Verification items for the finished model (mm, model axes). Face numbers are marked on the shaded views. Coordinates: 2 decimals unless noted, no trailing zeros. Write each loop counter-clockwise with the first axis right and the second up, starting at its lowest first coordinate (ties: lowest second). Pieces come first, ordered by that corner, then holes. Notation, with made-up numbers: M -23.5,65.25 L 32.5,65.25 A14 cw 32.5,80.25 Z; hole C -37.75,89 d9. An arc over 180 degrees is marked long. Answer in a Markdown table with one row per item.
Autodesk Fusion 360 part; units mm, degrees
sketch "Esboço1" plane through (0, 0, 0) normal (0, 1, 0) x (1, 0, 0)
  circle A0 centre (0, 0) radius 7.25
  dimension "d1" = 14.5
extrude "Extrusão1" add sketch "Esboço1" along normal blind 1
sketch "Esboço2" plane through (0, 1, 0) normal (0, 1, 0) x (-1, 0, 0)
  circle A0 centre (0, 0) radius 7.25
  circle A1 centre (0, 0) radius 6.8
  circle A2 centre (0, 0) radius 5.3
  dimension "d4" = 13.6
  dimension "d5" = -1.5
extrude "Extrusão2" add sketch "Esboço2" along normal blind 5 contours A1
sketch "Esboço3" plane through (0, 0, 0) normal (0, 0, 1) x (1, 0, 0)
  line L0 (6.8, 6) -> (6.8, 4)
  line L1 (6.8, 5) -> (6.9, 5)
  line L2 (6.9, 5) -> (6.8, 4)
  line L3 (6.9, 5) -> (6.8, 6)
revolve "Revolucionar1" add sketch "Esboço3" angle 360 about axis through (0, 1.75, 0) along (0, 1, 0)
fillet "Arredondamento1" radius 0.55 1 edges at (6.3398, 6, -2.459)
fillet "Arredondamento2" radius 0.55 1 edges at (4.9413, 6, 1.9166)
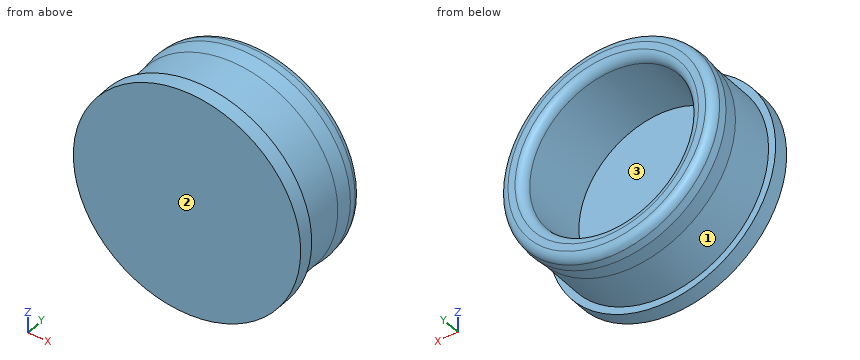
1) Sectioned sample at A-A (x = 0). Record the cut outline in (y, z), then the cut area to 3 significant figures.
Response values:
| item | result |
|---|---|
| outline | M 0,-7.25 L 1,-7.25 L 1,-6.8 L 4,-6.8 L 5,-6.9 L 5.5,-6.85 A0.55 ccw 6,-6.3 L 6,-5.85 A0.55 ccw 5.45,-5.3 L 1,-5.3 L 1,5.3 L 5.45,5.3 A0.55 ccw 6,5.85 L 6,6.3 A0.55 ccw 5.5,6.85 L 5,6.9 L 4,6.8 L 1,6.8 L 1,7.25 L 0,7.25 Z |
| area | 29.5 mm² |
2) Thickness scan on L1, parallel to Z at x = 0, y = 2.9; L2, parallel to Z at x = -3, y = 2; L3, parallel to Y at x = 0.75, z = -1.5. Record the ranges inside material, lowest first. Write a range as [from, to].
Response values:
| item | result |
|---|---|
| L1 | z = [-6.8, -5.3], [5.3, 6.8] |
| L2 | z = [-6.1, -4.37], [4.37, 6.1] |
| L3 | y = [0, 1] |
3) Depth check by flat-ended pin: pin 1 (2 mm diameter, centred on y = 4.5, z = -3.5, fed in from +X); pin 2 (4.5 mm diameter, centred on x = -0.5, z = 2, fed in from +Y); pin 3 (5.5 mm diameter, centred on x = 2.5, z = -1, fed in from +Y). Enter the tip coordinate at first touch or a pass-through.
Response values:
| item | result |
|---|---|
| pin 1 | stops at x = 6.39 |
| pin 2 | stops at y = 1 |
| pin 3 | stops at y = 5.82 |
4) Sectioned sample at B-B (z = 0). Record the cut outline in (x, y).
Response values:
| item | result |
|---|---|
| outline | M -7.25,0 L 7.25,0 L 7.25,1 L 6.8,1 L 6.8,4 L 6.9,5 L 6.85,5.5 A0.55 ccw 6.3,6 L 5.85,6 A0.55 ccw 5.3,5.45 L 5.3,1 L -5.3,1 L -5.3,5.45 A0.55 ccw -5.85,6 L -6.3,6 A0.55 ccw -6.85,5.5 L -6.9,5 L -6.8,4 L -6.8,1 L -7.25,1 Z |
5) Sectioned sample at C-C (y = 3.7). Record the cut outline in (x, z).
Response values:
| item | result |
|---|---|
| outline | C 0,0 d13.6; hole C 0,0 d10.6 |
6) Release check for a two-part mould opening along Y. For the marked faces 1, 2 and 3 record: +Y half, -Y half, draft (parallel to the pull), parting line (faces both ways), or undercut.
Response values:
| item | result |
|---|---|
| face 1 | undercut |
| face 2 | -Y half |
| face 3 | +Y half |
